Work out the finished part from the listing and answer in its coordinate system (mm). Round coordinates to 2 decimals unless told otherwise and drop trailing zeros. Write each loop counter-clockwise with the first axis right and the second up, starting at its lowest first coordinate (ties: lowest second). Pieces come first, ordered by that corner, then holes.
Autodesk Inventor part; units mm, degrees
ref_plane "YZ Plane" through (0, 0, 0) normal (1, 0, 0) x (0, 1, 0)
ref_plane "XZ Plane" through (0, 0, 0) normal (0, 1, 0) x (-1, 0, 0)
ref_plane "XY Plane" through (0, 0, 0) normal (0, 0, 1) x (1, 0, 0)
sketch "Sketch1" plane through (0, 0, 0) normal (0, 1, 0) x (-1, 0, 0)
  line L0 (0, 0) -> (76.2, 0)
  line L1 (76.2, 0) -> (76.2, -114.3)
  line L2 (76.2, -114.3) -> (0, -114.3)
  line L3 (0, -114.3) -> (0, 0)
  dimension "d0" = 76.2
  dimension "d1" = 114.3
extrude "Extrusion1" add sketch "Sketch1" along normal blind 3.175
hole "Hole1" at (-9.525, 3.175, -9.525) direction (0, -1, 0) diameter 6.35 depth 25.4 tip angle 118
hole "Hole2" at (-9.525, 3.175, -104.775) direction (0, -1, 0) diameter 6.35 depth 25.4 tip angle 118
hole "Hole3" at (-66.675, 3.175, -104.775) direction (0, -1, 0) diameter 6.35 depth 25.4 tip angle 118
hole "Hole4" at (-66.675, 3.175, -9.525) direction (0, -1, 0) diameter 6.35 depth 25.4 tip angle 118
hole "Hole5" at (-38.1, 3.175, -25.4) direction (0, -1, 0) diameter 28.575 depth 25.4 tip angle 118
properties part number "Back Gearbox Plate"
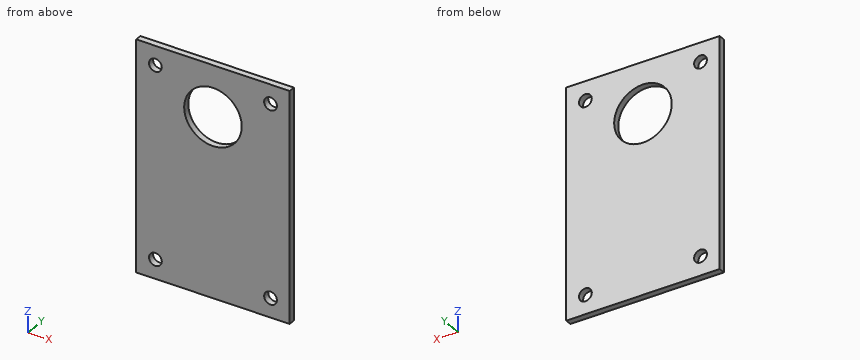
Q1. Find section A-A (z = -25.4). Determine the outline of the cut face in (x, y) (1 decimal), plus the area to 3 significant figures.
Q2. Given pin 1 (17 mm diameter, centred on x = -38.1, z = -25.4, fed in from -Y), flat-ended and moving along its own axis, determine where the tip first touches the part or whether it passes through.
Q3. Find section C-C (y = 1.35). Count the separate pieces of the cut face and the enclosed holes in it, plus the area to 3 significant figures.
Q4. Find section B-B (x = -38.1). Determine the outline of the cut face in (y, z) (1 decimal).
Q5. Find the intervals of material crossed by L1, parallel to Z at x = -38.1, y = 2.2; L2, parallel to X at y = 0.65, z = -106; L3, parallel to X at y = 0.7, z = -103.5, in increasing order.
Report:
1. outline: (-76.2, 0) - (-52.4, 0) - (-52.4, 3.2) - (-76.2, 3.2) - close; (-23.8, 0) - (0, 0) - (0, 3.2) - (-23.8, 3.2) - close
1. area: 151 mm2
2. pin 1: passes through
3. separate pieces: 1
3. enclosed holes: 5
3. area: 7,940 mm2
4. outline: (0, -114.3) - (3.2, -114.3) - (3.2, -39.7) - (0, -39.7) - close; (0, -11.1) - (3.2, -11.1) - (3.2, 0) - (0, 0) - close
5. L1: z = -114.3 to -39.69, -11.11 to 0
5. L2: x = -76.2 to -69.6, -63.75 to -12.45, -6.6 to 0
5. L3: x = -76.2 to -69.58, -63.77 to -12.43, -6.62 to 0
